Autodesk Inventor part; units mm, degrees
ref_plane "YZ Plane" through (0, 0, 0) normal (1, 0, 0) x (0, 1, 0)
ref_plane "XZ Plane" through (0, 0, 0) normal (0, 1, 0) x (-1, 0, 0)
ref_plane "XY Plane" through (0, 0, 0) normal (0, 0, 1) x (1, 0, 0)
sketch "Sketch1" plane through (0, 0, 0) normal (0, 1, 0) x (-1, 0, 0)
  line L0 (-15, -1.5) -> (15, -1.5)
  line L1 (15, 3.5) -> (15, 3.5)
  line L2 (15, 1.5) -> (-15, 1.5)
  line L3 (-15, 3.5) -> (-15, 3.5)
  line L4 (-15, -1.5) -> (15, 1.5) construction
  line L5 (15, -1.5) -> (-15, 1.5) construction
  circle A0 centre (13.5, 0) radius 1
  line L6 (-15, 1.5) -> (-15, -1.5)
  line L7 (15, 1.5) -> (15, -1.5)
  circle A1 centre (-13.5, 0) radius 1
  point P0 (0, 0)
  dimension "d0" = 3
  dimension "d1" = 30
  dimension "d3" = 2
  dimension "d6" = 1.5
  dimension "d8" = 1.5
  dimension "d13" = 2
  dimension "d14" = 1.5
  dimension "d15" = 1.5
extrude "Extrusion1" add sketch "Sketch1" along normal blind 5
properties part number "link"
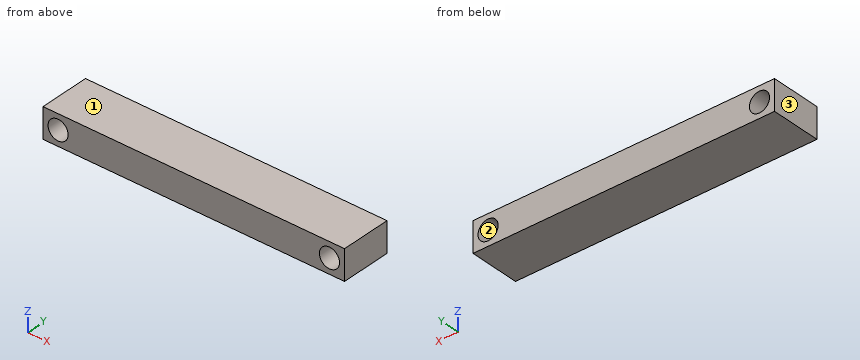
CAD build for the part. Positions are in the model's coordinates, mm. Face numbers are marked on the shaded views. Coordinates: 2 decimals unless noted, no trailing zeros. Write each loop counter-clockwise with the first axis right and the second up, starting at its lowest first coordinate (ties: lowest second). Pieces come first, ordered by that corner, then holes.
(1) Cut at A-A, the plane x = 13.5. List the corners of the cut face in (y, z), and give its area (3 significant figures).
(2) Cut at B-B, the plane y = 1.25. List the corners of the cut face in (x, z).
(3) Two-plate mould, pull along X, no slides. Class the marked faces 1, 2 and 3: +X half, -X half, draft (parallel to the pull), parting line (faces both ways), or undercut.
(4) Drill centre lines: probe 1 along X at (y, z) = (0.6, 0.05); probe 2 along Z at (x, y) = (13.5, 2); probe 3 along X at (y, z) = (3, 0.9). Where is each one in solid material? Low to high.
(5) Cut at C-C, the plane z = -0.75. List the corners of the cut face in (x, y), and give its area (3 significant figures).
Geometry says:
1. outline: (0, -1.5) - (5, -1.5) - (5, -1) - (0, -1) - close; (0, 1) - (5, 1) - (5, 1.5) - (0, 1.5) - close
1. area: 5.00 mm2
2. outline: (-15, -1.5) - (15, -1.5) - (15, 1.5) - (-15, 1.5) - close; hole circle Ø2 at (-13.5, 0); hole circle Ø2 at (13.5, 0)
3. face 1: draft
3. face 2: undercut
3. face 3: -X half
4. probe 1: x = -15 to -14.5, -12.5 to 12.5, 14.5 to 15
4. probe 2: z = -1.5 to -1, 1 to 1.5
4. probe 3: x = -15 to -13.94, -13.06 to 13.06, 13.94 to 15
5. outline: (-15, 0) - (-14.16, 0) - (-14.16, 5) - (-15, 5) - close; (-12.84, 0) - (12.84, 0) - (12.84, 5) - (-12.84, 5) - close; (14.16, 0) - (15, 0) - (15, 5) - (14.16, 5) - close
5. area: 137 mm2
